Input: part model. Units: mm. Frame: model coordinates. A direction names the side the tool comes from. Round coordinates to 2 decimals unless told otherwise and drop trailing zeros. Loops run counter-clockwise (first coordinate to the right, second up) from the corner with the lowest first, then second, coordinate; pieces in that order, holes last. Notation, with made-up numbers: M 24,-14.5 L 63,-14.5 A15 ccw 63,-0.5 Z; hole C 48,43.5 d1. An arc over 180 degrees is marked long. Use one line per item in the form item = value. Start each with the question number.
Q1. Section query B-B, the plane y = 32.5. Output: boundary loops of the cut face in (x, z), and give its area (3 significant figures).
Q2. First-contact query: P1, Ø12, axis at x = 106.5, z = -13.5, coming from the -Y side; P2, Ø1.5, axis at x = 49, y = 21, coming from the +Z side; P3, Ø1.5, axis at x = 120.5, y = 29.5, coming from the +Z side. Flat tips, straight axial feed; report the tip coordinate or a pass-through.
Q3. Section query C-C, the plane x = 109. Output: boundary loops of the cut face in (y, z), and give its area (3 significant figures).
Q4. Section query D-D, the plane x = 85. Output: boundary loops of the cut face in (y, z).
Q5. Mould query, pull axis X, two halves, no side actions, for faces 4 (the flat face through (163, 32, 0)), 5 (the cylindrical face through (135.32, 53.49, 27.38)), 6 (the cylindrical face through (160.535, 63.995, -16.381)), 7 (the flat face through (32, -0.3, -0.2)). Classes: pulls with the +X half, pulls with the -X half, needs draft (parallel to the pull), parting line crosses it, or undercut.
Q6. Access query for faces 1 (the flat face through (0, 32, 0)), 2 (the flat face through (80, -0.3, 0.2)), 3 (the cylindrical face through (16, 45, -30)). Directions: +Z, -Z, +X, -X, +Y, -Y. A direction counts if a zero-diameter tool reaches every point of the face in a straight line with its end or side. Return the directions, or none.
Q7. Section query A-A, the plane z = 0. Output: boundary loops of the cut face in (x, y), and give its area (3 significant figures).
Q8. Ray query, line 1 along X through (y, z) = (67, -2); line 2 along X through (y, z) = (41.5, -31.5); line 3 along X through (y, z) = (4, -21.5). Return the intervals inside material, ascending.
```python
from build123d import *


with BuildPart() as part:
    # Sketch1 → Revolve1 (revolve)
    with BuildSketch(Plane.XY, mode=Mode.PRIVATE) as revolve1_sk:
        with BuildLine():
            Line((0, 0), (32, 0))
            Line((32, 0), (32, -7.5))
            Line((32, -7.5), (80, -7.5))
            Line((80, -7.5), (80, 0))
            ThreePointArc((80, 0), (91, 11), (102, 0))
            Line((102, 0), (112, 0))
            Line((112, 0), (112, -2))
            Line((112, -2), (158, -2))
            Line((158, -2), (158, -3))
            Line((158, -3), (163, -3))
            Line((163, -3), (163, 32.5))
            Line((163, 32.5), (0, 32.5))
            Line((0, 32.5), (0, 0))
        make_face()
    revolve(revolve1_sk.sketch.rotate(Axis((163, 32.5, 0), (-1, 0, 0)), 270), axis=Axis((163, 32.5, 0), (-1, 0, 0)))


solid = part.part
```
Results found:
q1.outline = M 0,-32.5 L 32,-32.5 L 32,-40 L 80,-40 L 80,-32.5 A11 cw 102,-32.5 L 112,-32.5 L 112,-34.5 L 158,-34.5 L 158,-35.5 L 163,-35.5 L 163,35.5 L 158,35.5 L 158,34.5 L 112,34.5 L 112,32.5 L 102,32.5 A11 cw 80,32.5 L 80,40 L 32,40 L 32,32.5 L 0,32.5 Z
q1.area = 11,100 mm²
q2.P1 = -0.16
q2.P2 = 38.53
q2.P3 = 34.43
q3.outline = C 32.5,0 d65
q3.area = 3,320 mm²
q4.outline = C 32.5,0 d46.56
q5.face_4 = pulls with the +X half
q5.face_5 = undercut
q5.face_6 = needs draft
q5.face_7 = pulls with the -X half
q6.face_1 = +Z, -Z, -X, +Y, -Y
q6.face_2 = none
q6.face_3 = -X
q7.outline = M 0,0 L 32,0 L 32,-7.5 L 80,-7.5 L 80,0 A11 cw 102,0 L 112,0 L 112,-2 L 158,-2 L 158,-3 L 163,-3 L 163,68 L 158,68 L 158,67 L 112,67 L 112,65 L 102,65 A11 cw 80,65 L 80,72.5 L 32,72.5 L 32,65 L 0,65 Z
q7.area = 11,100 mm²
q8.line_1 = 32 to 80, 158 to 163
q8.line_2 = 32 to 80, 112 to 163
q8.line_3 = 32 to 80
